from build123d import *

# Parameters (mm, degrees)
BOX011_W      = 4
BOX011_H      = 80
BOX011_DEPTH  = 3
FILLET006_R   = 1
BOX010_W      = 30
BOX010_H      = 4
BOX010_DEPTH  = 3
FILLET007_R   = 1
BOX009_W      = 30
BOX009_H      = 4
BOX009_DEPTH  = 3
FILLET008_R   = 1
BOX008_W      = 30
BOX008_H      = 4
BOX008_DEPTH  = 3
FILLET009_R   = 1
BOX013_W      = 4
BOX013_H      = 80
BOX013_DEPTH  = 3
FILLET010_R   = 1
BOX012_W      = 30
BOX012_H      = 4
BOX012_DEPTH  = 3
FILLET005_R   = 1
BOX006_W      = 80
BOX006_H      = 10
BOX006_DEPTH  = 10
BOX007_W      = 80
BOX007_H      = 10
BOX007_DEPTH  = 10
FILLET004_1_R = 2
FILLET004_2_R = 1
BOX003_W      = 116
BOX003_H      = 179.5
BOX003_DEPTH  = 20
FILLET002_R   = 1.5
BOX002_W      = 120
BOX002_H      = 181
BOX002_DEPTH  = 12
FILLET003_R   = 1.5
BOX001_W      = 98
BOX001_H      = 173.5
BOX001_DEPTH  = 4
FILLET_R      = 1.5
BOX_W         = 120
BOX_H         = 181
BOX_DEPTH     = 4
FILLET001_R   = 1.5


with BuildPart() as fillet006:
    # Box011 → Box011 (new body)
    with BuildSketch(Plane(origin=(0, 50, 5), x_dir=(1, 0, 0), z_dir=(0, 0, 1))):
        with Locations((2, 40)):
            Rectangle(BOX011_W, BOX011_H)
    extrude(amount=BOX011_DEPTH)

    # Fillet006
    fillet006_edges = [fillet006.edges().sort_by_distance(p)[0] for p in [
        (0, 50, 6.5),
        (0, 130, 6.5),
    ]]
    fillet(fillet006_edges, radius=FILLET006_R)


with BuildPart() as fillet007:
    # Box010 → Box010 (new body)
    with BuildSketch(Plane(origin=(85, -3.5, 5), x_dir=(1, 0, 0), z_dir=(0, 0, 1))):
        with Locations((15, 2)):
            Rectangle(BOX010_W, BOX010_H)
    extrude(amount=BOX010_DEPTH)

    # Fillet007
    fillet007_edges = [fillet007.edges().sort_by_distance(p)[0] for p in [
        (85, -3.5, 6.5),
        (115, -3.5, 6.5),
    ]]
    fillet(fillet007_edges, radius=FILLET007_R)


with BuildPart() as fillet008:
    # Box009 → Box009 (new body)
    with BuildSketch(Plane(origin=(4, 180.5, 5), x_dir=(1, 0, 0), z_dir=(0, 0, 1))):
        with Locations((15, 2)):
            Rectangle(BOX009_W, BOX009_H)
    extrude(amount=BOX009_DEPTH)

    # Fillet008
    fillet008_edges = [fillet008.edges().sort_by_distance(p)[0] for p in [
        (4, 184.5, 6.5),
        (34, 184.5, 6.5),
    ]]
    fillet(fillet008_edges, radius=FILLET008_R)


with BuildPart() as fillet009:
    # Box008 → Box008 (new body)
    with BuildSketch(Plane(origin=(85, 180.5, 5), x_dir=(1, 0, 0), z_dir=(0, 0, 1))):
        with Locations((15, 2)):
            Rectangle(BOX008_W, BOX008_H)
    extrude(amount=BOX008_DEPTH)

    # Fillet009
    fillet009_edges = [fillet009.edges().sort_by_distance(p)[0] for p in [
        (85, 184.5, 6.5),
        (115, 184.5, 6.5),
    ]]
    fillet(fillet009_edges, radius=FILLET009_R)


with BuildPart() as fillet010:
    # Box013 → Box013 (new body)
    with BuildSketch(Plane(origin=(120.5, 50, 5), x_dir=(1, 0, 0), z_dir=(0, 0, 1))):
        with Locations((2, 40)):
            Rectangle(BOX013_W, BOX013_H)
    extrude(amount=BOX013_DEPTH)

    # Fillet010
    fillet010_edges = [fillet010.edges().sort_by_distance(p)[0] for p in [
        (124.5, 50, 6.5),
        (124.5, 130, 6.5),
    ]]
    fillet(fillet010_edges, radius=FILLET010_R)


with BuildPart() as fusion002:
    # Box012 → Box012 (new body)
    with BuildSketch(Plane(origin=(4, -3.5, 5), x_dir=(1, 0, 0), z_dir=(0, 0, 1))):
        with Locations((15, 2)):
            Rectangle(BOX012_W, BOX012_H)
    extrude(amount=BOX012_DEPTH)

    # Fillet005
    fillet005_edges = [fusion002.edges().sort_by_distance(p)[0] for p in [
        (4, -3.5, 6.5),
        (34, -3.5, 6.5),
    ]]
    fillet(fillet005_edges, radius=FILLET005_R)

    # Fusion002: union Fillet006, Fillet007, Fillet008, Fillet009, Fillet010
    add(fillet006.part)
    add(fillet007.part)
    add(fillet008.part)
    add(fillet009.part)
    add(fillet010.part)


with BuildPart() as fusion002_1:
    # Fusion002 placement: moved
    add(fusion002.part.moved(Location((0, 0, 5))))


with BuildPart() as cube006:
    # Box006 → Box006 (new body)
    with BuildSketch(Plane(origin=(15, -5, 0), x_dir=(1, 0, 0), z_dir=(0, 0, 1))):
        with Locations((40, 5)):
            Rectangle(BOX006_W, BOX006_H)
    extrude(amount=BOX006_DEPTH)


with BuildPart() as fillet004:
    # Box007 → Box007 (new body)
    with BuildSketch(Plane(origin=(15, 175, 0), x_dir=(1, 0, 0), z_dir=(0, 0, 1))):
        with Locations((40, 5)):
            Rectangle(BOX007_W, BOX007_H)
    extrude(amount=BOX007_DEPTH)

    # Fusion: union Cube006
    add(cube006.part)


with BuildPart() as fillet004_1:
    # Fusion placement: moved
    add(fillet004.part.moved(Location((0, 0, 13))))

    # Fillet004 1
    fillet004_1_edges = [fillet004_1.edges().sort_by_distance(p)[0] for p in [
        (15, 180, 13),
        (95, 180, 13),
    ]]
    fillet(fillet004_1_edges, radius=FILLET004_1_R)

    # Fillet004 2
    fillet004_2_edges = [fillet004_1.edges().sort_by_distance(p)[0] for p in [
        (15, 0, 13),
        (95, 0, 13),
    ]]
    fillet(fillet004_2_edges, radius=FILLET004_2_R)


with BuildPart() as fillet002:
    # Box003 → Box003 (new body)
    with BuildSketch(Plane(origin=(4, 0.75, 4), x_dir=(1, 0, 0), z_dir=(0, 0, 1))):
        with Locations((58, 89.75)):
            Rectangle(BOX003_W, BOX003_H)
    extrude(amount=BOX003_DEPTH)

    # Fillet002
    fillet002_edges = [fillet002.edges().sort_by_distance(p)[0] for p in [
        (4, 0.75, 14),
        (4, 180.25, 14),
        (120, 0.75, 14),
        (120, 180.25, 14),
    ]]
    fillet(fillet002_edges, radius=FILLET002_R)


with BuildPart() as cut002:
    # Box002 → Box002 (new body)
    with BuildSketch(Plane(origin=(2, 0, 4), x_dir=(1, 0, 0), z_dir=(0, 0, 1))):
        with Locations((60, 90.5)):
            Rectangle(BOX002_W, BOX002_H)
    extrude(amount=BOX002_DEPTH)

    # Fillet003
    fillet003_edges = [cut002.edges().sort_by_distance(p)[0] for p in [
        (2, 0, 10),
        (2, 181, 10),
        (122, 0, 10),
        (122, 181, 10),
    ]]
    fillet(fillet003_edges, radius=FILLET003_R)

    # Cut001: cut Fillet002
    add(fillet002.part, mode=Mode.SUBTRACT)

    # Cut002: cut Fillet004
    add(fillet004_1.part, mode=Mode.SUBTRACT)


with BuildPart() as fillet_body:
    # Box001 → Box001 (new body)
    with BuildSketch(Plane(origin=(7, 4, 0), x_dir=(1, 0, 0), z_dir=(0, 0, 1))):
        with Locations((49, 86.75)):
            Rectangle(BOX001_W, BOX001_H)
    extrude(amount=BOX001_DEPTH)

    # Fillet
    fillet_edges = [fillet_body.edges().sort_by_distance(p)[0] for p in [
        (7, 4, 2),
        (7, 177.5, 2),
        (105, 4, 2),
        (105, 177.5, 2),
    ]]
    fillet(fillet_edges, radius=FILLET_R)


with BuildPart() as fusion003:
    # Box → Box (new body)
    with BuildSketch(Plane(origin=(2, 0, 0), x_dir=(1, 0, 0), z_dir=(0, 0, 1))):
        with Locations((60, 90.5)):
            Rectangle(BOX_W, BOX_H)
    extrude(amount=BOX_DEPTH)

    # Fillet001
    fillet001_edges = [fusion003.edges().sort_by_distance(p)[0] for p in [
        (2, 0, 2),
        (2, 181, 2),
        (122, 0, 2),
        (122, 181, 2),
    ]]
    fillet(fillet001_edges, radius=FILLET001_R)

    # Cut: cut Fillet body
    add(fillet_body.part, mode=Mode.SUBTRACT)

    # Fusion001: union Cut002
    add(cut002.part)

    # Fusion003: union Fusion002
    add(fusion002_1.part)


solid = fusion003.part
The listing builds one solid part. Answer for the finished solid, in the listing's coordinates (mm). A direction names the side the tool comes from. Coordinates: 2 decimals unless noted, no trailing zeros. Loops run counter-clockwise (first coordinate to the right, second up) from the corner with the lowest first, then second, coordinate; pieces in that order, holes last. Notation, with made-up numbers: M -39.75,74.5 L -12.75,74.5 A27 cw -12.75,90.5 Z; hole C 67,46 d5. An arc over 180 degrees is marked long. Answer in a Markdown table with one row per item.
1) Determine the mould class of faces 5 (the flat face through (61, 0.75, 9)), 6 (the flat face through (7, 90, 2)), 7 (the flat face through (2, 89, 8)) for opening direction Y: released by +Y, released by -Y, zero draft, split by the parting line, or undercut.
Answers below:
| item | result |
|---|---|
| face 5 | undercut |
| face 6 | undercut |
| face 7 | zero draft |
2) Find section A-A (x = 78). Determine the outline of the cut face in (y, z).
Answers below:
| item | result |
|---|---|
| outline | M 0,0 L 4,0 L 4,4 L 0.75,4 L 0.75,13 L 0,13 Z; M 177.5,0 L 181,0 L 181,13 L 180.25,13 L 180.25,4 L 177.5,4 Z |
3) Find section D-D (x = 10.5). Determine the outline of the cut face in (y, z), then the cut area to 3 significant figures.
Answers below:
| item | result |
|---|---|
| outline | M -3.5,10 L 0,10 L 0,0 L 4,0 L 4,4 L 0.75,4 L 0.75,16 L 0,16 L 0,13 L -3.5,13 Z; M 177.5,0 L 181,0 L 181,10 L 184.5,10 L 184.5,13 L 181,13 L 181,16 L 180.25,16 L 180.25,4 L 177.5,4 Z |
| area | 69.0 mm^2 |
4) Given pin 1 (1.8 mm diameter, centred on x = 12.5, y = 182, fed in from -Z); pin 2 (1.5 mm diameter, centred on x = 24, z = 2.5, fed in from -Y); pin 3 (0.8 mm diameter, centred on y = 182.5, z = 11, fed in from +X); pin 4 (12 mm diameter, centred on x = 94.5, y = 46.5, fed in from +Z), each flat-ended and moving along its own axis, determine where each tip first touches the part or whether it passes through.
Answers below:
| item | result |
|---|---|
| pin 1 | z = 10 |
| pin 2 | y = 0 |
| pin 3 | x = 115 |
| pin 4 | through |
5) Find the intervals of material crossed by probe 1 along X at (y, z) = (82.5, 4.75); probe 2 along X at (y, z) = (158, 3.25); probe 3 along Y at (x, z) = (55, 9.5), in increasing order.
Answers below:
| item | result |
|---|---|
| probe 1 | 2 to 4, 120 to 122 |
| probe 2 | 2 to 7, 105 to 122 |
| probe 3 | 0 to 0.75, 180.25 to 181 |
6) Find section B-B (z = 6). Determine the outline of the cut face in (x, y), then the cut area to 3 significant figures.
Answers below:
| item | result |
|---|---|
| outline | M 2,1.5 A1.5 ccw 3.5,0 L 120.5,0 A1.5 ccw 122,1.5 L 122,179.5 A1.5 ccw 120.5,181 L 3.5,181 A1.5 ccw 2,179.5 Z; hole M 4,2.25 A1.5 ccw 5.5,0.75 L 118.5,0.75 A1.5 ccw 120,2.25 L 120,178.75 A1.5 ccw 118.5,180.25 L 5.5,180.25 A1.5 ccw 4,178.75 Z |
| area | 898 mm^2 |
7) Find section C-C (y = 91.5). Determine the outline of the cut face in (x, z).
Answers below:
| item | result |
|---|---|
| outline | M 0,10 L 2,10 L 2,0 L 7,0 L 7,4 L 4,4 L 4,16 L 2,16 L 2,13 L 0,13 Z; M 105,0 L 122,0 L 122,10 L 124.5,10 L 124.5,13 L 122,13 L 122,16 L 120,16 L 120,4 L 105,4 Z |
8) Which of the six approach directions +Z, -Z, +X, -X, +Y, -Y give full straight-line access (tool end or side, diameter ignored) to faces 1 (the flat face through (19, 183, 10)), 2 (the flat face through (55, 4, 2)), 3 (the flat face through (58.7, 180.5, 13)), 4 (the flat face through (109, 91, 4))?
Answers below:
| item | result |
|---|---|
| face 1 | -Z, +X, -X, +Y |
| face 2 | +Z, -Z |
| face 3 | +Z, +Y |
| face 4 | +Z |
